Could you check a few things on this model? Use its own coordinates, in mm. A direction names the side the tool comes from. Coordinates: 2 decimals unless noted, no trailing zeros. Loops run counter-clockwise (first coordinate to the right, second up) from the corner with the lowest first, then second, coordinate; pieces in that order, holes last.
from build123d import *

# Parameters (mm, degrees)
SKETCH1_R           = 2.525
SKETCH1_R_2         = 2.5
BOSS_EXTRUDE1_DEPTH = 6.35
SKETCH2_W           = 54
SKETCH2_H           = 54
CUT_EXTRUDE1_DEPTH  = 2.3
CUT_EXTRUDE2_DEPTH  = 2.3


with BuildPart() as part:
    # Sketch1 → Boss-Extrude1 (new body)
    with BuildSketch(Plane.XY):
        with BuildLine():
            Line((-47, 34), (47, 34))
            ThreePointArc((47, 34), (54.071067812, 31.071067812), (57, 24))
            Line((57, 24), (57, -24))
            ThreePointArc((57, -24), (54.071067812, -31.071067812), (47, -34))
            Line((47, -34), (-47, -34))
            ThreePointArc((-47, -34), (-54.071067812, -31.071067812), (-57, -24))
            Line((-57, -24), (-57, 24))
            ThreePointArc((-57, 24), (-54.071067812, 31.071067812), (-47, 34))
        make_face()
        with Locations((-47, -24)):
            Circle(SKETCH1_R, mode=Mode.SUBTRACT)
        with Locations((47, -24)):
            Circle(SKETCH1_R, mode=Mode.SUBTRACT)
        with Locations((47, 24)):
            Circle(SKETCH1_R, mode=Mode.SUBTRACT)
        with Locations((-47, 24)):
            Circle(SKETCH1_R, mode=Mode.SUBTRACT)
        with Locations((-17, 20)):
            Circle(SKETCH1_R, mode=Mode.SUBTRACT)
        with Locations((-17, -20)):
            Circle(SKETCH1_R, mode=Mode.SUBTRACT)
        with Locations((7, 20)):
            Circle(SKETCH1_R, mode=Mode.SUBTRACT)
        with Locations((7, -20)):
            Circle(SKETCH1_R, mode=Mode.SUBTRACT)
        with Locations((23, 0)):
            Circle(SKETCH1_R_2, mode=Mode.SUBTRACT)
    extrude(amount=BOSS_EXTRUDE1_DEPTH)

    # Sketch2 → Cut-Extrude1 (cut)
    with BuildSketch(Plane(origin=(0, 0, 0), x_dir=(-1, 0, 0), z_dir=(0, 0, -1))):
        with Locations((-1, 0)):
            Rectangle(SKETCH2_W, SKETCH2_H)
    extrude(amount=-CUT_EXTRUDE1_DEPTH, mode=Mode.SUBTRACT)

    # Sketch3 → Cut-Extrude2 (cut)
    with BuildSketch(Plane(origin=(0, 0, 2.3), x_dir=(-1, 0, 0), z_dir=(0, 0, -1))):
        with BuildLine():
            Line((-22.483177153, 27), (-22.483177153, 21.483177153))
            Line((-22.483177153, 21.483177153), (-28, 21.483177153))
            ThreePointArc((-28, 21.483177153), (-28.127559597, 22.485277608), (-28.502102661, 23.423464298))
            ThreePointArc((-28.502102661, 23.423464298), (-28, 27), (-24.423464298, 27.502102661))
            ThreePointArc((-24.423464298, 27.502102661), (-23.485277608, 27.127559597), (-22.483177153, 27))
        make_face()
        with BuildLine():
            Line((20.483177153, 21.483177153), (26, 21.483177153))
            ThreePointArc((26, 21.483177153), (26.127559597, 22.485277608), (26.502102661, 23.423464298))
            ThreePointArc((26.502102661, 23.423464298), (26, 27), (22.423464298, 27.502102661))
            ThreePointArc((22.423464298, 27.502102661), (21.485277608, 27.127559597), (20.483177153, 27))
            Line((20.483177153, 27), (20.483177153, 21.483177153))
        make_face()
        with BuildLine():
            Line((20.483177153, -27), (20.483177153, -21.483177153))
            Line((20.483177153, -21.483177153), (26, -21.483177153))
            ThreePointArc((26, -21.483177153), (26.127559597, -22.485277608), (26.502102661, -23.423464298))
            ThreePointArc((26.502102661, -23.423464298), (26, -27), (22.423464298, -27.502102661))
            ThreePointArc((22.423464298, -27.502102661), (21.485277608, -27.127559597), (20.483177153, -27))
        make_face()
        with BuildLine():
            Line((-22.483177153, -21.483177153), (-28, -21.483177153))
            ThreePointArc((-28, -21.483177153), (-28.127559597, -22.485277608), (-28.502102661, -23.423464298))
            ThreePointArc((-28.502102661, -23.423464298), (-28, -27), (-24.423464298, -27.502102661))
            ThreePointArc((-24.423464298, -27.502102661), (-23.485277608, -27.127559597), (-22.483177153, -27))
            Line((-22.483177153, -27), (-22.483177153, -21.483177153))
        make_face()
    extrude(amount=CUT_EXTRUDE2_DEPTH, mode=Mode.SUBTRACT)


solid = part.part
1) Imagine slicing it at C-C on z = 4.25. State how many separate pieces and enclosed holes the cut face has, plus the area to 3 significant figures.
2) Imagine slicing it at A-A on x = 7. List the corners of the cut face in (y, z) for me (3 decimals), plus the area to 3 significant figures.
3) Will this pin go through, and if not, where does the flat tip stop? pin 1 (6 mm diameter, centred on x = -2.5, y = -4, fed in from -Z).
4) Imagine slicing it at B-B on y = 0. List the corners of the cut face in (x, z) for me, plus the area to 3 significant figures.
5) For faces 1 (the cylindrical face through (53.99, 31.15, 3.13)), 2 (the cylindrical face through (28, -27, 1)), which set-ups out of +Z, -Z, +X, -X, +Y, -Y let a thin tool reach every point of the face, with its end or its side?
6) Imagine slicing it at D-D on y = 20. List the corners of the cut face in (x, z) for me (3 decimals).
7) If I drill on L1, parallel to Y at x = -17, z = 3.2 (3 decimals); L2, parallel to X at y = 20, z = 5.45 (3 decimals); L3, parallel to Y at x = -8, z = 0.5, over which ranges is the centre line in solid material (lowest first)?
8) We'd pull the mould along Y, two halves only. Please class faces 3 (the flat face through (1, -34, 3)), 4 (the flat face through (1, -30, 0)), 5 (the flat face through (1, -27, 1)): released by +Y, released by -Y, zero draft, split by the parting line, or undercut.
Solved:
1. separate pieces: 1
1. enclosed holes: 9
1. area: 7,490 mm2
2. outline: (-34, 0) - (-27, 0) - (-27, 2.3) - (-22.525, 2.3) - (-22.525, 6.35) - (-34, 6.35) - close; (-17.475, 2.3) - (17.475, 2.3) - (17.475, 6.35) - (-17.475, 6.35) - close; (22.525, 2.3) - (27, 2.3) - (27, 0) - (34, 0) - (34, 6.35) - (22.525, 6.35) - close
2. area: 267 mm2
3. pin 1: stops at z = 2.3
4. outline: (-57, 0) - (-26, 0) - (-26, 2.3) - (20.5, 2.3) - (20.5, 6.35) - (-57, 6.35) - close; (25.5, 2.3) - (28, 2.3) - (28, 0) - (57, 0) - (57, 6.35) - (25.5, 6.35) - close
4. area: 579 mm2
5. face 1: +Z, -Z, +X, +Y
5. face 2: -Z
6. outline: (-57, 0) - (-26, 0) - (-26, 2.3) - (-19.525, 2.3) - (-19.525, 6.35) - (-57, 6.35) - close; (-14.475, 2.3) - (4.475, 2.3) - (4.475, 6.35) - (-14.475, 6.35) - close; (9.525, 2.3) - (28, 2.3) - (28, 0) - (57, 0) - (57, 6.35) - (9.525, 6.35) - close
7. L1: y = -34 to -22.525, -17.475 to 17.475, 22.525 to 34
7. L2: x = -57 to -19.525, -14.475 to 4.475, 9.525 to 57
7. L3: y = -34 to -27, 27 to 34
8. face 3: released by -Y
8. face 4: zero draft
8. face 5: undercut
